from build123d import *

# Parameters (mm, degrees)
PAD_DEPTH       = 15
PAD001_DEPTH    = 14
SKETCH002_R     = 4.02
HOLE_DEPTH      = 26.635776
POCKET_DEPTH    = 21.635776
POCKET001_DEPTH = 8


with BuildPart() as body:
    # Sketch → Pad (new body)
    with BuildSketch(Plane.XZ):
        Polygon((30, 7.667262), (11.667262, 26), (0, 14.332738), (0, 0), (30, 0), align=None)
    extrude(amount=PAD_DEPTH)

    # Sketch001 → Pad001 (join)
    with BuildSketch(Plane.XY):
        with BuildLine():
            ThreePointArc((0, -27.02), (4.02, -23), (0, -18.98))
            Line((0, -18.98), (0, -15))
            Line((0, -15), (15.491933, -15))
            ThreePointArc((15.491933, -15), (12.329656, -16.55051), (11.61895, -20))
            ThreePointArc((0, -35), (9.486833, -30.348469), (11.61895, -20))
            Line((0, -35), (0, -27.02))
        make_face()
    extrude(amount=PAD001_DEPTH)

    # Sketch002 (on DatumPlane) → Hole (cut, through all)
    with BuildSketch(Plane(origin=(18.833631, 0, 18.833631), x_dir=(-0.707107, 0, 0.707107), z_dir=(0.707107, 0, 0.707107))):
        with Locations((0.634776, 0)):
            Circle(SKETCH002_R)
    extrude(amount=-HOLE_DEPTH, mode=Mode.SUBTRACT)

    # Sketch003 (on DatumPlane) → Pocket (cut, through all)
    with BuildSketch(Plane(origin=(15.298097, 0, 15.298097), x_dir=(-0.707107, 0, 0.707107), z_dir=(0.707107, 0, 0.707107))):
        Polygon((7.384776, 3.897114), (0.634776, 7.794229), (-6.115224, 3.897114), (-6.115224, -3.897114), (0.634776, -7.794229), (7.384776, -3.897114), align=None)
    extrude(amount=-POCKET_DEPTH, mode=Mode.SUBTRACT)

    # Sketch004 (on Face13 of Pocket) → Pocket001 (cut)
    with BuildSketch(Plane(origin=(0, 0, 14), x_dir=(-1, 0, 0), z_dir=(0, 0, 1))):
        Polygon((3.897114, 29.75), (-3.897114, 29.75), (-7.794229, 23), (-3.897114, 16.25), (3.897114, 16.25), (7.794229, 23), align=None)
    extrude(amount=-POCKET001_DEPTH, mode=Mode.SUBTRACT)


with BuildPart() as part_mirroring:
    # Part__Mirroring: instance of Body
    add(body.part.mirror(Plane(origin=(0, 0, 0), x_dir=(0, -1, 0), z_dir=(1, 0, 0))))


with BuildPart() as part_mirroring002:
    # Part__Mirroring002: instance of Part__Mirroring
    add(part_mirroring.part.mirror(Plane(origin=(0, 0, 0), x_dir=(1, 0, 0), z_dir=(0, 1, 0))))


with BuildPart() as fusion:
    # Part__Mirroring001: instance of Body
    add(body.part.mirror(Plane(origin=(0, 0, 0), x_dir=(1, 0, 0), z_dir=(0, 1, 0))))

    # Fusion: union Body, Part__Mirroring002, Part__Mirroring
    add(body.part)
    add(part_mirroring002.part)
    add(part_mirroring.part)


solid = fusion.part
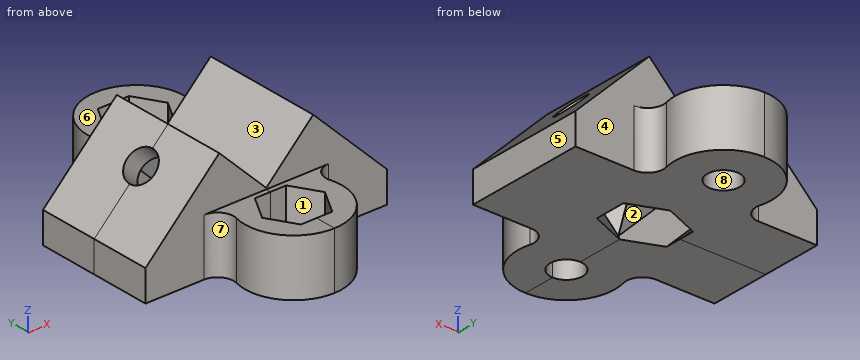
Source: CAD feature listing. Evaluate the final solid. Frame: model axes, mm. Face numbers are marked on the shaded views. A direction names the side the tool comes from. Round coordinates to 2 decimals unless told otherwise and drop trailing zeros. Loops run counter-clockwise (first coordinate to the right, second up) from the corner with the lowest first, then second, coordinate; pieces in that order, holes last. Notation, with made-up numbers: (11.5, 18.25) - (58.5, 18.25) arc R14 cw to (58.5, 22.25) - close; hole circle Ø1 at (-35.5, 89). An arc over 180 degrees is marked (long way). Write item = value, one per line. Start each with the question number.
(1) Section query D-D, the plane x = -23.5. Output: boundary loops of the cut face in (y, z).
(2) Ray query, line 1 along X through (y, z) = (-5, 15.75); line 2 along X through (y, z) = (3, 14.25); line 3 along X through (y, z) = (23, 4.45). Return the intervals inside material, ascending. Write a range as from..to.
(3) Section query A-A, the plane y = -26. Output: boundary loops of the cut face in (x, z).
(4) Section query C-C, the plane z = 9. State how many separate pieces and enclosed holes the cut face has, plus the area to 3 significant figures.
(5) Pin query (flat end, axial travel): pin 1 (4 mm diameter, centred on x = 1.5, y = -0.5, fed in from +Z); pin 2 (4 mm diameter, centred on x = -3.5, y = 21, fed in from +Z); pin 3 (6 mm diameter, centred on x = 3.5, y = -20.5, fed in from +Z); pin 4 (4.5 mm diameter, centred on x = -1, z = 10.5, fed in from +Y). Return the tip coordinate at first contact, or that it passes through.
(6) Section query B-B, the plane y = 9.5. Output: boundary loops of the cut face in (x, z).
(7) Pull-direction query (X, two-part tool) for the marked faces 6, 7 and 8; classes: +X half, -X half, draft (parallel to the pull), parting line (faces both ways), or undercut.
(8) Set-up query: the marked faces 1, 2, 3, 4 and 5. Return all of +Z, -Z, +X, -X, +Y, -Y with unobstructed straight access to the full face (end or side cutting, diameter ignored); none if empty.
Conclusion:
q1.outline = (-15, 0) - (15, 0) - (15, 14.17) - (-15, 14.17) - close
q2.line_1 = -21.92..-14.85, -8.01..-1.42, 1.42..8.01, 14.85..21.92
q2.line_2 = -23.42..-17.14, -3.81..3.81, 17.14..23.42
q2.line_3 = -12..-4.02, 4.02..12
q3.outline = (-11.62, 0) - (-2.68, 0) - (-2.68, 6) - (-6.06, 6) - (-6.06, 14) - (-11.62, 14) - close; (2.68, 0) - (11.62, 0) - (11.62, 14) - (6.06, 14) - (6.06, 6) - (2.68, 6) - close
q4.separate_pieces = 1
q4.enclosed_holes = 3
q4.area = 1,820 mm2
q5.pin_1 = 17.83
q5.pin_2 = 6
q5.pin_3 = 14
q5.pin_4 = 35
q6.outline = (-30, 0) - (30, 0) - (30, 7.67) - (11.67, 26) - (0, 14.33) - (-11.67, 26) - (-30, 7.67) - close
q7.face_6 = draft
q7.face_7 = -X half
q7.face_8 = undercut
q8.face_1 = +Z
q8.face_2 = none
q8.face_3 = +Z, +Y, -Y
q8.face_4 = +Z, +Y
q8.face_5 = +Z, -Z, +X, +Y, -Y
